from build123d import *

# Parameters (mm, degrees)
BOSS_EXTRUDE1_DEPTH              = 500
F_0_15_44_5_DIAMETER_HOLE1_D     = 44.5
F_0_15_44_5_DIAMETER_HOLE1_DEPTH = 2


with BuildPart() as part:
    # Sketch1 → Boss-Extrude1 (new, symmetric)
    with BuildSketch(Plane(origin=(0, 0, 0), x_dir=(0, 0, -1), z_dir=(1, 0, 0))):
        with BuildLine():
            Line((-50.85, -27.5), (50.85, -27.5))
            ThreePointArc((50.85, -27.5), (52.264213562, -26.914213562), (52.85, -25.5))
            Line((52.85, -25.5), (52.85, 25.5))
            ThreePointArc((52.85, 25.5), (52.264213562, 26.914213562), (50.85, 27.5))
            Line((50.85, 27.5), (-50.85, 27.5))
            ThreePointArc((-50.85, 27.5), (-52.264213562, 26.914213562), (-52.85, 25.5))
            Line((-52.85, 25.5), (-52.85, -25.5))
            ThreePointArc((-52.85, -25.5), (-52.264213562, -26.914213562), (-50.85, -27.5))
        make_face()
        with BuildLine():
            Line((-48.85, 25.5), (48.85, 25.5))
            ThreePointArc((48.85, 25.5), (50.264213562, 24.914213562), (50.85, 23.5))
            Line((50.85, 23.5), (50.85, -23.5))
            ThreePointArc((50.85, -23.5), (50.264213562, -24.914213562), (48.85, -25.5))
            Line((48.85, -25.5), (-48.85, -25.5))
            ThreePointArc((-48.85, -25.5), (-50.264213562, -24.914213562), (-50.85, -23.5))
            Line((-50.85, -23.5), (-50.85, 23.5))
            ThreePointArc((-50.85, 23.5), (-50.264213562, 24.914213562), (-48.85, 25.5))
        make_face(mode=Mode.SUBTRACT)
    extrude(amount=BOSS_EXTRUDE1_DEPTH, both=True)

    # Ø0.15 (44.5) Diameter Hole1
    with Locations(Plane(origin=(0, 27.5, 0), x_dir=(1, 0, 0), z_dir=(0, 1, 0))):
        with Locations((-444.5, 0), (-317.5, 0), (-190.5, 0), (-63.5, 0), (63.5, 0), (190.5, 0), (317.5, 0), (444.5, 0)):
            Hole(F_0_15_44_5_DIAMETER_HOLE1_D / 2, depth=F_0_15_44_5_DIAMETER_HOLE1_DEPTH)


solid = part.part
Work out the finished part from the listing and answer in its coordinate system (mm). A direction names the side the tool comes from. Give positions to 0.01 mm unless a question says otherwise; leave off trailing zeros. Order: outer loops, then holes, each group sorted by start corner. A loop starts at its lowest first (then second) coordinate and runs counter-clockwise, first axis right, second up. Notation, with made-up numbers: (84, 19.5) -> (96, 19.5) arc R35 cw to (96, 58.5) -> close; hole circle Ø7 at (57, 12.25). An arc over 180 degrees is marked (long way). One line per item, written item: value.
Item 1: Find section B-B, the plane z = -33.5. Give the vertices of the cut face in (x, y), plus the area to 3 significant figures.
Answer sheet:
outline: (-500, -27.5) -> (500, -27.5) -> (500, -25.5) -> (-500, -25.5) -> close; (-500, 25.5) -> (500, 25.5) -> (500, 27.5) -> (-500, 27.5) -> close
area: 4,000 mm²
Item 2: Find section A-A, the plane y = 8.5. Give the vertices of the cut face in (x, z), plus the area to 3 significant figures.
Answer sheet:
outline: (-500, -52.85) -> (500, -52.85) -> (500, -50.85) -> (-500, -50.85) -> close; (-500, 50.85) -> (500, 50.85) -> (500, 52.85) -> (-500, 52.85) -> close
area: 4,000 mm²
Item 3: A tool of negligible diameter and unlimited length cuts with its end or side. For faces 5 (the flat face through (7, 0, 52.85)), 6 (the cylindrical face through (466.73, 26.49, -0.98)), 7 (the flat face through (7, -25.5, -1)), from which of +Z, -Z, +X, -X, +Y, -Y can it reach the whole face along a straight path? Write none if from no direction.
Answer sheet:
face 5: +Z, +X, -X, +Y, -Y
face 6: +Y
face 7: +X, -X
Item 4: Find section D-D, the plane x = -68. Give the vertices of the cut face in (y, z).
Answer sheet:
outline: (-27.5, -50.85) arc R2 ccw to (-25.5, -52.85) -> (25.5, -52.85) arc R2 ccw to (27.5, -50.85) -> (27.5, -21.79) -> (25.5, -21.79) -> (25.5, -48.85) arc R2 cw to (23.5, -50.85) -> (-23.5, -50.85) arc R2 cw to (-25.5, -48.85) -> (-25.5, 48.85) arc R2 cw to (-23.5, 50.85) -> (23.5, 50.85) arc R2 cw to (25.5, 48.85) -> (25.5, 21.79) -> (27.5, 21.79) -> (27.5, 50.85) arc R2 ccw to (25.5, 52.85) -> (-25.5, 52.85) arc R2 ccw to (-27.5, 50.85) -> close
Item 5: Straight lines are drawn through the part: probe 1 along Y at (x, z) = (-389, -33.5); probe 2 along Z at (x, y) = (194, -11.5); probe 3 along Z at (x, y) = (317, 26). For each, find the intervals that lie inside material, in ascending order.
Answer sheet:
probe 1: -27.5 to -25.5, 25.5 to 27.5
probe 2: -52.85 to -50.85, 50.85 to 52.85
probe 3: -52.79 to -22.24, 22.24 to 52.79
Item 6: A flat-ended cylindrical pin translates along its axis: P1, Ø2, axis at x = -184, z = -15, coming from the +Y side. Find the tip coordinate at first contact, or state that the pin passes through.
Answer sheet:
P1: y = -25.5
Item 7: Find section C-C, the plane x = -399.5. Give the vertices of the cut face in (y, z).
Answer sheet:
outline: (-27.5, -50.85) arc R2 ccw to (-25.5, -52.85) -> (25.5, -52.85) arc R2 ccw to (27.5, -50.85) -> (27.5, 50.85) arc R2 ccw to (25.5, 52.85) -> (-25.5, 52.85) arc R2 ccw to (-27.5, 50.85) -> close; hole (-25.5, -48.85) arc R2 ccw to (-23.5, -50.85) -> (23.5, -50.85) arc R2 ccw to (25.5, -48.85) -> (25.5, 48.85) arc R2 ccw to (23.5, 50.85) -> (-23.5, 50.85) arc R2 ccw to (-25.5, 48.85) -> close
Item 8: Determine the mould class of faces 1 (the cylindrical face through (-295.27, 26.49, -0.98)), 2 (the cylindrical face through (339.73, 26.49, -0.98)), 3 (the flat face through (500, 27, 16)), 4 (the flat face through (7, -27.5, 1)) for opening direction X: released by +X, released by -X, zero draft, split by the parting line, or undercut.
Answer sheet:
face 1: undercut
face 2: undercut
face 3: released by +X
face 4: zero draft
